Could you check a few things on this model? Use its own coordinates, in mm. Give positions to 0.01 mm unless a question says otherwise; leave off trailing zeros. Order: outer loops, then holes, each group sorted by start corner. A loop starts at its lowest first (then second) coordinate and runs counter-clockwise, first axis right, second up. Notation, with made-up numbers: (20, 53) -> (47, 53) arc R19 ccw to (47, 65) -> close; hole circle Ø11 at (58.25, -14). An arc over 180 degrees is marked (long way). Answer as CSV lines item,"result". Start each with the question number.
(1) I need wall thicknesses on L1, parallel to X at y = 19.05, z = 1.5 (3 decimals); L2, parallel to Y at x = 0, z = 1.15; L3, parallel to X at y = 95.25, z = 1.15. Which ranges of each line are inside material? Lowest first, please.
(2) I want a section at C-C (y = -50.5). Please give me the cut outline in (x, z) (3 decimals), plus the area to 3 significant figures.
(3) Will this pin go through, and if not, where does the flat tip stop? pin 1 Ø4 at (x, y) = (-66.675, 44.45) entering from -Z.
(4) I want a section at A-A (x = -90). Please give me the cut outline in (y, z) (3 decimals).
(5) I want a section at B-B (z = 0.5). Please give me the cut outline in (x, y) (3 decimals), plus the area to 3 significant figures.
```python
from build123d import *

# Parameters (mm, degrees)
F1_DEPTH = 3.175
F2_D     = 4.4958
F3_D     = 4.4958
F4_D     = 4.4958
F5_D     = 4.4958
F6_D     = 4.4958


with BuildPart() as f1:
    # F0 (on Top) → F1 (new body)
    with BuildSketch(Plane.XY):
        with BuildLine():
            Line((-107.95, -69.85), (-107.95, -107.95))
            Line((-107.95, -107.95), (107.95, -107.95))
            Line((107.95, -107.95), (107.95, -69.85))
            Line((107.95, -69.85), (82.55, -69.85))
            ThreePointArc((82.55, -69.85), (80.3049359697, -68.9200640303), (79.375, -66.675))
            Line((79.375, -66.675), (79.375, 66.675))
            ThreePointArc((79.375, 66.675), (80.3049359697, 68.9200640303), (82.55, 69.85))
            Line((82.55, 69.85), (107.95, 69.85))
            Line((107.95, 69.85), (107.95, 107.95))
            Line((107.95, 107.95), (-107.95, 107.95))
            Line((-107.95, 107.95), (-107.95, 69.85))
            Line((-107.95, 69.85), (-82.55, 69.85))
            ThreePointArc((-82.55, 69.85), (-80.3049359697, 68.9200640303), (-79.375, 66.675))
            Line((-79.375, 66.675), (-79.375, -66.675))
            ThreePointArc((-79.375, -66.675), (-80.3049359697, -68.9200640303), (-82.55, -69.85))
            Line((-82.55, -69.85), (-107.95, -69.85))
        make_face()
    extrude(amount=F1_DEPTH)

    # F2 (through all)
    with Locations(Plane(origin=(0, 0, 0), x_dir=(1, 0, 0), z_dir=(0, 0, -1))):
        with Locations((0, 0)):
            Hole(F2_D / 2)

    # F3 (through all)
    with Locations(Plane(origin=(0, 0, 0), x_dir=(1, 0, 0), z_dir=(0, 0, -1))):
        with Locations((-66.675, -95.25)):
            Hole(F3_D / 2)

    # F4 (through all)
    with Locations(Plane(origin=(0, 0, 0), x_dir=(1, 0, 0), z_dir=(0, 0, -1))):
        with Locations((-66.675, -69.85)):
            Hole(F4_D / 2)

    # F5 (through all)
    with Locations(Plane(origin=(0, 0, 0), x_dir=(1, 0, 0), z_dir=(0, 0, -1))):
        with Locations((-66.675, -44.45)):
            Hole(F5_D / 2)

    # F6 (through all)
    with Locations(Plane(origin=(0, 0, 0), x_dir=(1, 0, 0), z_dir=(0, 0, -1))):
        with Locations((-66.675, -19.05)):
            Hole(F6_D / 2)


solid = f1.part
```
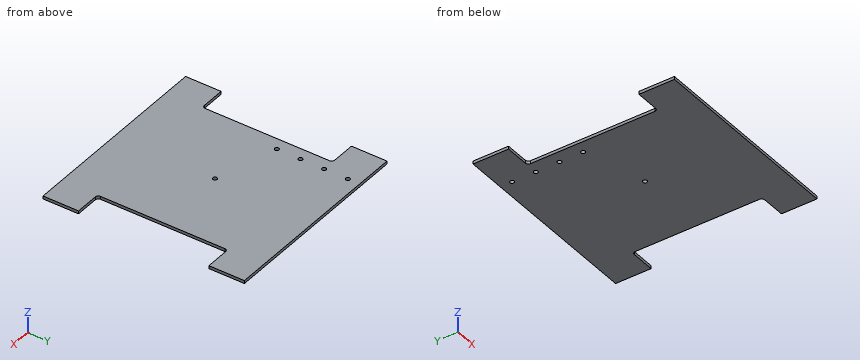
Final values:
1,L1,"-79.375 to -68.923, -64.427 to 79.375"
1,L2,"-107.95 to -2.25, 2.25 to 107.95"
1,L3,"-107.95 to -68.92, -64.43 to 107.95"
2,outline,"(-79.375, 0) -> (79.375, 0) -> (79.375, 3.175) -> (-79.375, 3.175) -> close"
2,area,"504 mm²"
3,pin 1,"through"
4,outline,"(-107.95, 0) -> (-69.85, 0) -> (-69.85, 3.175) -> (-107.95, 3.175) -> close; (69.85, 0) -> (107.95, 0) -> (107.95, 3.175) -> (69.85, 3.175) -> close"
5,outline,"(-107.95, -107.95) -> (107.95, -107.95) -> (107.95, -69.85) -> (82.55, -69.85) arc R3.175 cw to (79.375, -66.675) -> (79.375, 66.675) arc R3.175 cw to (82.55, 69.85) -> (107.95, 69.85) -> (107.95, 107.95) -> (-107.95, 107.95) -> (-107.95, 69.85) -> (-82.55, 69.85) arc R3.175 cw to (-79.375, 66.675) -> (-79.375, -66.675) arc R3.175 cw to (-82.55, -69.85) -> (-107.95, -69.85) -> close; hole circle Ø4.496 at (-66.675, 19.05); hole circle Ø4.496 at (-66.675, 44.45); hole circle Ø4.496 at (-66.675, 69.85); hole circle Ø4.496 at (-66.675, 95.25); hole circle Ø4.496 at (0, 0)"
5,area,"38,600 mm²"
